Part print with two shaded views. Sizes in mm from the minimum x, y, z corner. A direction names the side the tool comes from. Round coordinates to 2 decimals unless told otherwise and drop trailing zeros. Write each loop counter-clockwise with the first axis right and the second up, starting at its lowest first coordinate (ties: lowest second). Pieces come first, ordered by that corner, then holes. Notation, with made-up numbers: (15, -37.5) -> (65, -37.5) arc R23 ccw to (65, -0.5) -> close; hole circle Ø8 at (21.5, 14.5). An arc over 180 degrees is marked (long way). Answer as CSV lines item,"result".
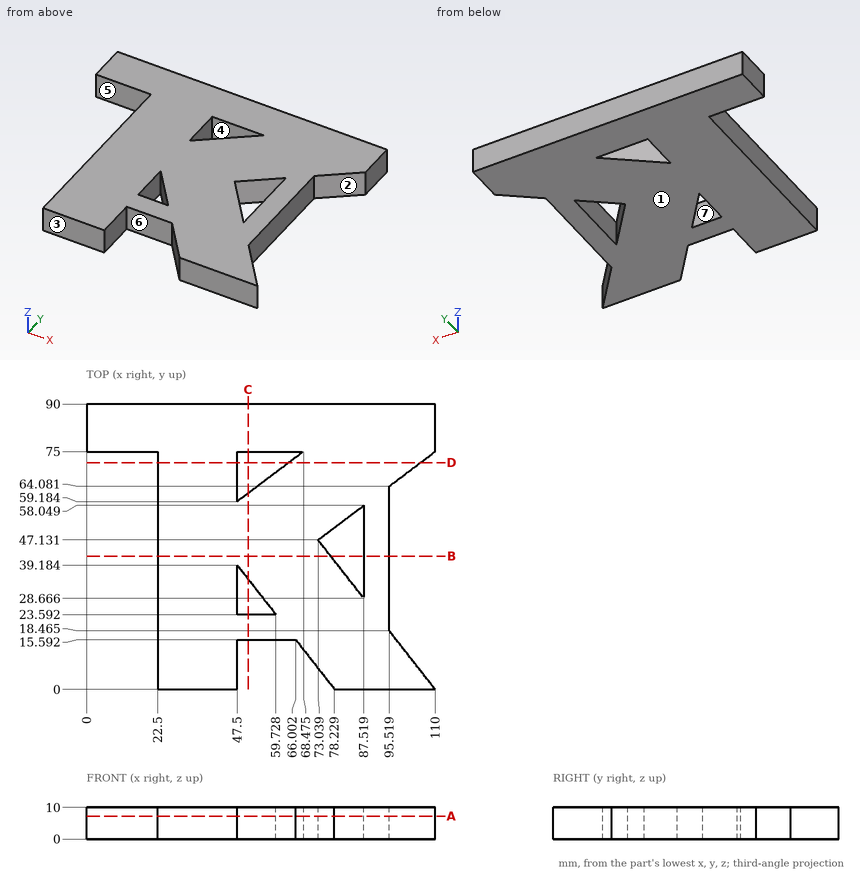
1. Probe line 1 along Y through (x, z) = (15.5, 8); line 2 along X through (y, z) = (37.5, 4.75); line 3 along X through (y, z) = (49, 3.5) (1 decimal). List the from-to ranges inside material, lowest first.
Results found:
line 1,"y = 75 to 90"
line 2,"x = 22.5 to 47.5, 48.82 to 80.59, 87.52 to 95.52"
line 3,"x = 22.5 to 75.5, 87.5 to 95.5"
2. Mould opens along Y. For the marked faces 1, 2, 3 and 4 say: +Y half, -Y half, draft (parallel to the pull), parting line (faces both ways), or undercut.
Results found:
face 1,"draft"
face 2,"undercut"
face 3,"-Y half"
face 4,"undercut"
3. Cut at B-B, the plane y = 42. Write the cut outline in (x, z).
Results found:
outline,"(22.5, 0) -> (77.06, 0) -> (77.06, 10) -> (22.5, 10) -> close; (87.52, 0) -> (95.52, 0) -> (95.52, 10) -> (87.52, 10) -> close"
4. Drop flat-ended pins along their axis: pin 1 Ø3 at (x, z) = (61.5, 7) entering from -Y; pin 2 Ø3 at (y, z) = (28.5, 5.5) entering from +X; pin 3 Ø5 at (x, z) = (10, 7) entering from -Y. Give the stop position or say it passes through.
Results found:
pin 1,"stops at y = 15.59"
pin 2,"stops at x = 95.52"
pin 3,"stops at y = 75"
5. Which spindle directions (+Z, -Z, +X, -X, +Y, -Y) get a long thin tool onto all of the face, cutting with end or side? Do the marked faces 5, 6 and 7. Say none if no direction does.
Results found:
face 5,"+Z, -Z, -X, -Y"
face 6,"+Z, -Z, -Y"
face 7,"+Z, -Z"
6. Cut at A-A, the plane z = 7.25. Count the separate pieces of the cut face and the enclosed holes in it, then the cut area to 3 significant figures.
Results found:
separate pieces,"1"
enclosed holes,"3"
area,"6,480 mm2"
7. Cut at D-D, the plane y = 71.5. Write the cut outline in (x, z), then the cut area to 3 significant figures.
Results found:
outline,"(22.5, 0) -> (47.5, 0) -> (47.5, 10) -> (22.5, 10) -> close; (63.83, 0) -> (105.36, 0) -> (105.36, 10) -> (63.83, 10) -> close"
area,"665 mm2"
8. Cut at C-C, the plane x = 51. Write the cut outline in (y, z).
Results found:
outline,"(15.59, 0) -> (23.59, 0) -> (23.59, 10) -> (15.59, 10) -> close; (34.72, 0) -> (61.82, 0) -> (61.82, 10) -> (34.72, 10) -> close; (75, 0) -> (90, 0) -> (90, 10) -> (75, 10) -> close"
